```python
from build123d import *

# Parameters (mm, degrees)
SKETCH_1_W                 = 240
SKETCH_1_H                 = 146
SKETCH_1_R                 = 11
SKETCH_1_R_2               = 3
SKETCH_1_R_3               = 3.5
EXTRUDE_1_DEPTH            = 2
HOLE_WIZARD_M22_AT_2_COUNT = 2
HOLE_WIZARD_M22_AT_2_PITCH = 224
HOLE_WIZARD_M22_AT_3_COUNT = 2
HOLE_WIZARD_M22_AT_3_PITCH = 258.99034731
HOLE_WIZARD_M22_AT_4_COUNT = 2
HOLE_WIZARD_M22_AT_4_PITCH = 130


with BuildPart() as part:
    # Эскиз1 → Бобышка-Вытянуть1 (new body)
    with BuildSketch(Plane.XY):
        with Locations((120, 73)):
            Rectangle(SKETCH_1_W, SKETCH_1_H)
        with Locations((79.765350749, 26)):
            Circle(SKETCH_1_R, mode=Mode.SUBTRACT)
        with Locations((48.515350749, 26)):
            Circle(SKETCH_1_R_2, mode=Mode.SUBTRACT)
        with Locations((167, 73)):
            Circle(SKETCH_1_R_2, mode=Mode.SUBTRACT)
        with Locations((90.832011317, 93)):
            Circle(SKETCH_1_R_2, mode=Mode.SUBTRACT)
        with Locations((40, 68.913299822)):
            Circle(SKETCH_1_R_2, mode=Mode.SUBTRACT)
        with Locations((20, 138)):
            Circle(SKETCH_1_R_3, mode=Mode.SUBTRACT)
        with Locations((220, 138)):
            Circle(SKETCH_1_R_3, mode=Mode.SUBTRACT)
        with Locations((220, 8)):
            Circle(SKETCH_1_R_3, mode=Mode.SUBTRACT)
        with Locations((20, 8)):
            Circle(SKETCH_1_R_3, mode=Mode.SUBTRACT)
    extrude(amount=EXTRUDE_1_DEPTH)

    # Эскиз7 → Зенковка для винта с полупотайной головкой M22 (revolve, cut)
    with BuildSketch(Plane(origin=(8, 138, 2), x_dir=(0, -1, 0), z_dir=(1, 0, 0))):
        Polygon((0, 0), (0, 2), (1.2, 2), (1.2, 1), (2.2, 0), align=None)
    hole_wizard_m22 = revolve(axis=Axis((8, 138, 8.35), (0, 0, -1)), mode=Mode.SUBTRACT)

    # Зенковка для винта с полупотайной головкой M22 at 2: Зенковка для винта с полупотайной головкой M22 ×2
    with Locations(*[(i * HOLE_WIZARD_M22_AT_2_PITCH, 0, 0) for i in range(1, HOLE_WIZARD_M22_AT_2_COUNT)]):
        add(hole_wizard_m22, mode=Mode.SUBTRACT)

    # Зенковка для винта с полупотайной головкой M22 at 3: Зенковка для винта с полупотайной головкой M22 ×2
    with Locations(*[Vector(0.864897099, -0.501949209, 0) * (i * HOLE_WIZARD_M22_AT_3_PITCH) for i in range(1, HOLE_WIZARD_M22_AT_3_COUNT)]):
        add(hole_wizard_m22, mode=Mode.SUBTRACT)

    # Зенковка для винта с полупотайной головкой M22 at 4: Зенковка для винта с полупотайной головкой M22 ×2
    with Locations(*[(0, -i * HOLE_WIZARD_M22_AT_4_PITCH, 0) for i in range(1, HOLE_WIZARD_M22_AT_4_COUNT)]):
        add(hole_wizard_m22, mode=Mode.SUBTRACT)


solid = part.part
```
CAD build for the part. Positions are in the model's coordinates, mm. Round coordinates to 2 decimals unless told otherwise and drop trailing zeros. Loops run counter-clockwise (first coordinate to the right, second up) from the corner with the lowest first, then second, coordinate; pieces in that order, holes last. Notation, with made-up numbers: (-31, 53) - (26, 53) arc R27 cw to (26, 71) - close; hole circle Ø7 at (77.25, -8.5). An arc over 180 degrees is marked (long way). Return JSON: item names as keys, results as strings. Group by question number.
Q1. Flat gauge pin, fed straight in: pin 1 Ø5 at (x, y) = (90.83, 93) entering from -Z. Where does the tip first touch, or does it go through?
Q2. Band-saw the part on A-A on x = 220. Give the cut face in (y, z).
Q3. Drill centre lines: line 1 along Y through (x, z) = (220, 0.45); line 2 along X through (y, z) = (138, 0.5); line 3 along X through (y, z) = (10, 0.45). Where is each one in solid material? Low to high. Write a range as [from, to].
Q4. Band-saw the part on B-B on y = 93. Give the cut face in (x, z), plus the area to 3 significant figures.
Q5. Band-saw the part on D-D on z = 1.4. Give the number of separate pieces and of enclosed holes in the cut face, plus the area to 3 significant figures.
Q6. Band-saw the part on C-C on x = 167. Give the cut face in (y, z), plus the area to 3 significant figures.
Q7. Two-plate mould, pull along Y, no slides. Class faces 1 (the face through (118, 74, 0)), 2 (the face through (92.22, 90.34, 0.99)): +Y half, -Y half, draft (parallel to the pull), parting line (faces both ways), or undercut.
Solutions:
{
 "1": {"pin 1": "passes through"},
 "2": {"outline": "(0, 0) - (4.5, 0) - (4.5, 2) - (0, 2) - close; (11.5, 0) - (134.5, 0) - (134.5, 2) - (11.5, 2) - close; (141.5, 0) - (146, 0) - (146, 2) - (141.5, 2) - close"},
 "3": {"line 1": "y = [0, 4.5], [11.5, 134.5], [141.5, 146]", "line 2": "x = [0, 6.8], [9.2, 16.5], [23.5, 216.5], [223.5, 230.8], [233.2, 240]", "line 3": "x = [0, 17.13], [22.87, 217.13], [222.87, 240]"},
 "4": {"outline": "(0, 0) - (87.83, 0) - (87.83, 2) - (0, 2) - close; (93.83, 0) - (240, 0) - (240, 2) - (93.83, 2) - close", "area": "468 mm^2"},
 "5": {"separate pieces": "1", "enclosed holes": "13", "area": "34,400 mm^2"},
 "6": {"outline": "(0, 0) - (70, 0) - (70, 2) - (0, 2) - close; (76, 0) - (146, 0) - (146, 2) - (76, 2) - close", "area": "280 mm^2"},
 "7": {"face 1": "draft", "face 2": "undercut"}
}
